```python
from build123d import *

# Parameters (mm, degrees)
F1_DEPTH = 12.7


with BuildPart() as f1:
    # F0 (on Front) → F1 (new body, symmetric)
    with BuildSketch(Plane.XZ):
        Polygon((-37.203092, 0), (0, 0), (8.250058, 0), (8.250058, -17.90107), (44.986166, -17.90107), (44.986166, 13.853871), (0, 35.957802), (-37.203092, 35.957802), align=None)
        Polygon((-22.259591, 8.872705), (-22.259591, 23.816206), (10.117996, 18.83504), (31.910602, 6.38212), (35.335157, -9.184027), (25.061497, -9.184027), (12.297258, 8.872705), align=None, mode=Mode.SUBTRACT)
    extrude(amount=F1_DEPTH, both=True)


solid = f1.part
```
Source: CAD feature listing. Evaluate the final solid. Frame: model axes, mm. A direction names the side the tool comes from. Give positions to 0.01 mm unless a question says otherwise; leave off trailing zeros. Order: outer loops, then holes, each group sorted by start corner. A loop starts at its lowest first (then second) coordinate and runs counter-clockwise, first axis right, second up.
(1) Contact query for flat-ended pins moving along their axis: P1, Ø4, axis at x = 14.5, y = 0.5, coming from the +Z side; P2, Ø11.5, axis at x = 29, y = -3, coming from the +Z side; P3, Ø1.5, axis at x = -4.5, y = 3, coming from the -Z side. Output: stop coordinate, or through.
(2) Pull-direction query (Z, two-part tool) for faces 4 (the face through (18.769, -0.178, -0.282)), 5 (the face through (26, 0, -17.901)), 6 (the face through (-37.203, 0, 18)); classes: +Z half, -Z half, draft (parallel to the pull), parting line (faces both ways), or undercut.
(3) Section query D-D (x = -29). Return the cut outline in (y, z), plus the area to 3 significant figures.
(4) Section query A-A (y = -4.75). Return the cut outline in (x, z).
(5) Access query for faces 1 (the face through (20.862, -0.178, 12.696)), 2 (the face through (22.81, -0.18, 24.75)), 3 (the face through (-15, 0, 0)). Directions: +Z, -Z, +X, -X, +Y, -Y. A direction counts if a zero-diameter tool reaches every point of the face in a straight line with its end or side. Return the directions, or none.
(6) Material intervals for line 1 along Z through (x, y) = (-4, 6.5); line 2 along X through (y, z) = (-10, -0.5); line 3 along Z through (x, y) = (19.5, -6.25), sorted ascending.
(7) Section query B-B (z = 16). Return the cut outline in (x, y), plus the area to 3 significant figures.
(8) Section query C-C (x = -2.5). Return the cut outline in (y, z).
Outcome:
1. P1: stops at z = 29.82
1. P2: stops at z = 24.53
1. P3: stops at z = 0
2. face 4: undercut
2. face 5: -Z half
2. face 6: draft
3. outline: (-12.7, 0) - (12.7, 0) - (12.7, 35.96) - (-12.7, 35.96) - close
3. area: 913 mm2
4. outline: (-37.2, 0) - (8.25, 0) - (8.25, -17.9) - (44.99, -17.9) - (44.99, 13.85) - (0, 35.96) - (-37.2, 35.96) - close; hole (-22.26, 8.87) - (12.3, 8.87) - (25.06, -9.18) - (35.34, -9.18) - (31.91, 6.38) - (10.12, 18.84) - (-22.26, 23.82) - close
5. face 1: +Y, -Y
5. face 2: +Z, +X, +Y, -Y
5. face 3: -Z, -X, +Y, -Y
6. line 1: z = 0 to 8.87, 21.01 to 35.96
6. line 2: x = 8.25 to 18.92, 33.42 to 44.99
6. line 3: z = -17.9 to -1.32, 13.47 to 26.38
7. outline: (-37.2, -12.7) - (-22.26, -12.7) - (-22.26, 12.7) - (-37.2, 12.7) - close; (15.08, -12.7) - (40.62, -12.7) - (40.62, 12.7) - (15.08, 12.7) - close
7. area: 1,030 mm2
8. outline: (-12.7, 0) - (12.7, 0) - (12.7, 8.87) - (-12.7, 8.87) - close; (-12.7, 20.78) - (12.7, 20.78) - (12.7, 35.96) - (-12.7, 35.96) - close
